from build123d import *

# Parameters (mm, degrees)
SKETCH_1_R          = 0.9
SKETCH_1_W          = 31.5
SKETCH_1_H          = 49.5
EXTRUDE_1_DEPTH     = 4
SKETCH_2_W          = 80
SKETCH_2_H          = 22.5
EXTRUDE_2_DEPTH     = 15
SKETCH_3_R          = 0.9
CUT_EXTRUDE_1_DEPTH = 20
SKETCH_4_R          = 0.9
CUT_EXTRUDE_2_DEPTH = 20
SKETCH_6_W          = 72
SKETCH_6_H          = 11
CUT_EXTRUDE_3_DEPTH = 18.5
SKETCH_7_R          = 1.4
CUT_EXTRUDE_5_DEPTH = 8


with BuildPart() as part:
    # 스케치1 → 보스-돌출1 (new body)
    with BuildSketch(Plane.XZ):
        with BuildLine():
            Line((45, -52.5), (45, 67.5))
            Line((45, 67.5), (-35, 67.5))
            Line((-35, 67.5), (-35, -52.5))
            Line((-35, -52.5), (-22.946377225, -52.5))
            ThreePointArc((-22.946377225, -52.5), (5, -41.5), (32.946377225, -52.5))
            Line((32.946377225, -52.5), (45, -52.5))
        make_face()
        with Locations((-28.975, -41.744959148)):
            Circle(SKETCH_1_R, mode=Mode.SUBTRACT)
        with Locations((-28.975, -6.5)):
            Circle(SKETCH_1_R, mode=Mode.SUBTRACT)
        with Locations((-32.75, 65.25)):
            Circle(SKETCH_1_R, mode=Mode.SUBTRACT)
        with Locations((5, 65.25)):
            Circle(SKETCH_1_R, mode=Mode.SUBTRACT)
        with Locations((42.75, 65.25)):
            Circle(SKETCH_1_R, mode=Mode.SUBTRACT)
        with Locations((38.975, -6.5)):
            Circle(SKETCH_1_R, mode=Mode.SUBTRACT)
        with Locations((38.975, -41.744959148)):
            Circle(SKETCH_1_R, mode=Mode.SUBTRACT)
        with Locations((5, 16)):
            Rectangle(SKETCH_1_W, SKETCH_1_H, mode=Mode.SUBTRACT)
    extrude(amount=-EXTRUDE_1_DEPTH)

    # 스케치2 → 보스-돌출2 (add)
    with BuildSketch(Plane(origin=(0, 4, 0), x_dir=(1, 0, 0), z_dir=(0, 1, 0))):
        with Locations((5, -56.25)):
            Rectangle(SKETCH_2_W, SKETCH_2_H)
        with BuildLine():
            Line((45, 32.5), (-35, 32.5))
            Line((-35, 32.5), (-35, 52.5))
            Line((-35, 52.5), (-22.946377225, 52.5))
            ThreePointArc((-22.946377225, 52.5), (5, 41.5), (32.946377225, 52.5))
            Line((32.946377225, 52.5), (45, 52.5))
            Line((45, 52.5), (45, 32.5))
        make_face()
    extrude(amount=EXTRUDE_2_DEPTH)

    # 스케치3 → 컷-돌출1 (cut, through all)
    with BuildSketch(Plane(origin=(0, 19, 0), x_dir=(1, 0, 0), z_dir=(0, 1, 0))):
        with Locations((38.975, 42.5)):
            Circle(SKETCH_3_R)
        with Locations((-28.975, 42.5)):
            Circle(SKETCH_3_R)
    extrude(amount=-CUT_EXTRUDE_1_DEPTH, mode=Mode.SUBTRACT)

    # 스케치4 → 컷-돌출2 (cut, through all)
    with BuildSketch(Plane.XZ):
        with Locations((42.75, 65.25)):
            Circle(SKETCH_4_R)
        with Locations((5, 65.25)):
            Circle(SKETCH_4_R)
        with Locations((-32.75, 65.25)):
            Circle(SKETCH_4_R)
    extrude(amount=-CUT_EXTRUDE_2_DEPTH, mode=Mode.SUBTRACT)

    # 스케치6 → 컷-돌출3 (cut)
    with BuildSketch(Plane(origin=(0, 0, 45), x_dir=(-1, 0, 0), z_dir=(0, 0, -1))):
        with Locations((-5, 9.5)):
            Rectangle(SKETCH_6_W, SKETCH_6_H)
    extrude(amount=-CUT_EXTRUDE_3_DEPTH, mode=Mode.SUBTRACT)

    # 스케치7 → 컷-돌출5 (cut)
    with BuildSketch(Plane(origin=(0, 19, 0), x_dir=(1, 0, 0), z_dir=(0, 1, 0))):
        with Locations((21.25, 37.5)):
            Circle(SKETCH_7_R)
        with Locations((-11.25, 37.5)):
            Circle(SKETCH_7_R)
    extrude(amount=-CUT_EXTRUDE_5_DEPTH, mode=Mode.SUBTRACT)


solid = part.part
Model file for the job. Use its own axes, mm. A direction names the side the tool comes from. Round coordinates to 2 decimals unless told otherwise and drop trailing zeros. Order: outer loops, then holes, each group sorted by start corner. A loop starts at its lowest first (then second) coordinate and runs counter-clockwise, first axis right, second up.
(1) Band-saw the part on C-C (x = 11.5). List the corners of the cut face in (y, z).
(2) Band-saw the part on A-A (y = 12.75). Give the number of separate pieces and of enclosed holes in the cut face, then the cut area to 3 significant figures.
(3) Pull direction Z, two halves, no side cores. Call faces 1 (the face through (22, 4, 16)), 2 (the face through (-35, 3, 22)), 3 (the face through (4.6, 9.4, -41.5)): released by +Z, released by -Z, zero draft, split by the parting line, or undercut.
(4) 3-axis set-ups, long thin cutter, end or side, ignore diameter. For faces 4 (the face through (6, 10, 63.5)), 5 (the face through (5, 2, 40.75)), 6 (the face through (6, 11, -32.5)), 7 (the face through (-11.43, 15.06, -38.89)): which of +Z, -Z, +X, -X, +Y, -Y reach the whole face in a straight line?
(5) Band-saw the part on D-D (x = 36). List the corners of the cut face in (y, z), then the cut area to 3 significant figures.
(6) Drill centre lines: line 1 (X direction, y = 5.25, z = 65.25); line 2 (X direction, y = 12, z = 60.5); line 3 (Z direction, x = -2, y = 14.25). Where is each one in solid material? Low to high.
(7) Band-saw the part on B-B (z = -0.5). List the corners of the cut face in (x, y).
(8) Pin check, flat tips, straight feed: pin 1 (5.5 mm diameter, centred on x = 6.5, y = 8, fed in from -Z); pin 2 (10 mm diameter, centred on x = -22.5, z = 37, fed in from +Y); pin 3 (3 mm diameter, centred on x = -11, z = -38, fed in from +Y); pin 4 (0.6 mm diameter, centred on x = 38.5, z = -41.5, fed in from -Y). Stop position of each tip, or through.
Verdict:
1. outline: (0, -42.02) - (19, -42.02) - (19, -32.5) - (4, -32.5) - (4, -8.75) - (0, -8.75) - close; (0, 40.75) - (4, 40.75) - (4, 63.5) - (15, 63.5) - (15, 45) - (19, 45) - (19, 67.5) - (0, 67.5) - close
2. separate pieces: 2
2. enclosed holes: 7
2. area: 1,620 mm2
3. face 1: undercut
3. face 2: zero draft
3. face 3: released by -Z
4. face 4: none
4. face 5: +Y, -Y
4. face 6: +X, -X, +Y
4. face 7: +Y
5. outline: (0, -52.5) - (19, -52.5) - (19, -32.5) - (4, -32.5) - (4, 63.5) - (15, 63.5) - (15, 45) - (19, 45) - (19, 67.5) - (0, 67.5) - close
5. area: 914 mm2
6. line 1: x = -35 to -33.65, -31.85 to 4.1, 5.9 to 41.85, 43.65 to 45
6. line 2: x = -35 to -31, 41 to 45
6. line 3: z = -42.1 to -32.5, 63.5 to 67.5
7. outline: (-35, 0) - (-10.75, 0) - (-10.75, 4) - (-35, 4) - close; (20.75, 0) - (45, 0) - (45, 4) - (20.75, 4) - close
8. pin 1: stops at z = -41.72
8. pin 2: stops at y = 4
8. pin 3: stops at y = 19
8. pin 4: stops at y = 4
